from build123d import *
from build123d.topology import SkipClean

# Parameters (mm, degrees)
SKETCH1_R           = 158.75
BOSS_EXTRUDE1_DEPTH = 45.974


with BuildPart() as part:
    # Sketch1 → Boss-Extrude1 (new body)
    with BuildSketch(Plane.XY):
        Circle(SKETCH1_R)
        with BuildLine():
            Line((-3.175, 88.6419075), (-3.175, 21.997045256))
            ThreePointArc((-3.175, 21.997045256), (-11.1125, 19.247414599), (-17.4625, 13.748153285))
            Line((-17.4625, 13.748153285), (-75.178643735, 47.070584407))
            ThreePointArc((-75.178643735, 47.070584407), (-80.796594988, 53.906629613), (-79.935272493, 62.712934961))
            ThreePointArc((-79.935272493, 62.712934961), (-50.8, 87.988181024), (-14.343358575, 100.582444118))
            ThreePointArc((-14.343358575, 100.582444118), (-6.286213183, 96.925218605), (-3.175, 88.6419075))
        make_face(mode=Mode.SUBTRACT)
        with BuildLine():
            ThreePointArc((-94.278631069, 37.869509157), (-87.082808171, 43.018588992), (-78.353643735, 41.571323093))
            Line((-78.353643735, 41.571323093), (-20.6375, 8.248891971))
            ThreePointArc((-20.6375, 8.248891971), (-22.225, 0), (-20.6375, -8.248891971))
            Line((-20.6375, -8.248891971), (-78.353643735, -41.571323093))
            ThreePointArc((-78.353643735, -41.571323093), (-87.082808171, -43.018588992), (-94.278631069, -37.869509157))
            ThreePointArc((-94.278631069, -37.869509157), (-101.6, 0), (-94.278631069, 37.869509157))
        make_face(mode=Mode.SUBTRACT)
        with BuildLine():
            ThreePointArc((-79.935272493, -62.712934961), (-80.796594988, -53.906629613), (-75.178643735, -47.070584407))
            Line((-75.178643735, -47.070584407), (-17.4625, -13.748153285))
            ThreePointArc((-17.4625, -13.748153285), (-11.1125, -19.247414599), (-3.175, -21.997045256))
            Line((-3.175, -21.997045256), (-3.175, -88.6419075))
            ThreePointArc((-3.175, -88.6419075), (-6.286213183, -96.925218605), (-14.343358575, -100.582444118))
            ThreePointArc((-14.343358575, -100.582444118), (-50.8, -87.988181024), (-79.935272493, -62.712934961))
        make_face(mode=Mode.SUBTRACT)
        with BuildLine():
            ThreePointArc((14.343358575, -100.582444118), (6.286213183, -96.925218605), (3.175, -88.6419075))
            Line((3.175, -88.6419075), (3.175, -21.997045256))
            ThreePointArc((3.175, -21.997045256), (11.1125, -19.247414599), (17.4625, -13.748153285))
            Line((17.4625, -13.748153285), (75.178643735, -47.070584407))
            ThreePointArc((75.178643735, -47.070584407), (80.796594988, -53.906629613), (79.935272493, -62.712934961))
            ThreePointArc((79.935272493, -62.712934961), (50.8, -87.988181024), (14.343358575, -100.582444118))
        make_face(mode=Mode.SUBTRACT)
        with BuildLine():
            ThreePointArc((94.278631069, -37.869509157), (87.082808171, -43.018588992), (78.353643735, -41.571323093))
            Line((78.353643735, -41.571323093), (20.6375, -8.248891971))
            ThreePointArc((20.6375, -8.248891971), (22.225, 0), (20.6375, 8.248891971))
            Line((20.6375, 8.248891971), (78.353643735, 41.571323093))
            ThreePointArc((78.353643735, 41.571323093), (87.082808171, 43.018588992), (94.278631069, 37.869509157))
            ThreePointArc((94.278631069, 37.869509157), (101.6, 0), (94.278631069, -37.869509157))
        make_face(mode=Mode.SUBTRACT)
        with BuildLine():
            ThreePointArc((79.935272493, 62.712934961), (80.796594988, 53.906629613), (75.178643735, 47.070584407))
            Line((75.178643735, 47.070584407), (17.4625, 13.748153285))
            ThreePointArc((17.4625, 13.748153285), (11.1125, 19.247414599), (3.175, 21.997045256))
            Line((3.175, 21.997045256), (3.175, 89.414085543))
            ThreePointArc((3.175, 89.414085543), (6.554659404, 97.202784714), (14.343358575, 100.582444118))
            ThreePointArc((14.343358575, 100.582444118), (50.8, 87.988181024), (79.935272493, 62.712934961))
        make_face(mode=Mode.SUBTRACT)
        with BuildLine():
            Line((9.059069904, -8.896430657), (6.189629933, -7.239758718))
            ThreePointArc((6.189629933, -7.239758718), (-8.248891971, 4.7625), (9.364629933, -1.740497404))
            Line((9.364629933, -1.740497404), (12.234069904, -3.397169343))
            Line((12.234069904, -3.397169343), (9.059069904, -8.896430657))
        make_face(mode=Mode.SUBTRACT)
    extrude(amount=BOSS_EXTRUDE1_DEPTH)

    # Sketch2 → Cut-Revolve1 (revolve, cut)
    with BuildSketch(Plane(origin=(0, 0, 0), x_dir=(1, 0, 0), z_dir=(0, 1, 0))):
        with BuildLine():
            Line((158.75, -45.974), (158.75, -22.987))
            ThreePointArc((158.75, -22.987), (157.121901144, -34.91676007), (152.356680652, -45.974))
            Line((152.356680652, -45.974), (158.75, -45.974))
        make_face()
        with BuildLine():
            Line((158.75, 0), (152.356680652, 0))
            ThreePointArc((152.356680652, 0), (157.121901144, -11.05723993), (158.75, -22.987))
            Line((158.75, -22.987), (158.75, 0))
        make_face()
    revolve(axis=Axis((0, 0, 0), (0, 0, -1)), mode=Mode.SUBTRACT)

    # Sketch2_6 → Revolve2 (revolve)
    with SkipClean():  # the faces are left unmerged after this step: merging them gives an invalid solid
        with BuildSketch(Plane(origin=(0, 0, 0), x_dir=(1, 0, 0), z_dir=(0, 1, 0))):
            with BuildLine():
                ThreePointArc((146.05, -54.124579906), (149.439969417, -50.232386632), (152.356680652, -45.974))
                Line((152.356680652, -45.974), (114.256680652, -45.974))
                Line((114.256680652, -45.974), (146.05, -54.124579906))
            make_face()
            with BuildLine():
                ThreePointArc((152.356680652, 0), (149.439969417, 4.258386632), (146.05, 8.150579906))
                Line((146.05, 8.150579906), (114.256680652, 0))
                Line((114.256680652, 0), (152.356680652, 0))
            make_face()
        revolve(axis=Axis((0, 0, 0), (0, 0, -1)))


solid = part.part
Design review of the part built by this model. Coordinates are the model's own, in mm. A direction names the side the tool comes from. Round coordinates to 2 decimals unless told otherwise and drop trailing zeros. Use one line per item in the form item = value. Start each with the question number.
Q1. We need section A-A on x = 44. State how many separate pieces and enclosed holes the cut face has, then the cut area to 3 significant figures.
Q2. Machinability: for faces 1 (the face through (-9, 9, 45.974)), 2 (the face through (-49.9, 25.143, 22.665)), 3 (the face through (-25.103, 113.047, -0.396)), which of the approach directions +Z, -Z, +X, -X, +Y, -Y give a long, thin tool a straight path to every point of the face, cutting with its end or side? Answer none if there is none.
Q3. For pin 1 Ø8 at (x, y) = (35, -103) entering from +Z; pin 2 Ø6 at (x, z) = (-66, 20) entering from +Y; pin 3 Ø10 at (x, z) = (118.5, 30.5) entering from +Y; pin 4 Ø3 at (x, y) = (-73, -34.5) entering from -Z, all flat-tipped, find the tip position at first contact; note any pin that passes through.
Q4. Wall thickness on line 1 along Y through (x, z) = (-77, 7); line 2 along X through (y, z) = (-36.5, 24.5) (3 decimals); line 3 along X through (y, z) = (-48, 35) (3 decimals): over which ranges is each line inside the solid? List them lowest first. Write a range as [from, to].
Calculated:
q1.separate_pieces = 4
q1.enclosed_holes = 0
q1.area = 6,750 mm²
q2.face_1 = +Z
q2.face_2 = +Z, -Z
q2.face_3 = -Z
q3.pin_1 = 45.97
q3.pin_2 = 145.62
q3.pin_3 = 110.2
q3.pin_4 = through
q4.line_1 = [-135.42, -66.28], [-48.28, -40.79], [40.79, 48.28], [66.28, 135.42]
q4.line_2 = [-154.471, -94.817], [-69.57, -56.87], [-3.175, 3.175], [56.87, 69.57], [94.817, 154.471]
q4.line_3 = [-149.586, -76.644], [-3.175, 3.175], [76.644, 149.586]
